Work out the finished part from the listing and answer in its coordinate system (mm). Face numbers are marked on the shaded views. A direction names the side the tool comes from. Give positions to 0.01 mm unless a question says otherwise; leave off trailing zeros. Order: outer loops, then holes, each group sorted by start corner. A loop starts at its lowest first (then second) coordinate and runs counter-clockwise, first axis right, second up. Notation, with made-up numbers: (17, 59.25) - (57, 59.25) arc R29 ccw to (57, 98.25) - close; hole circle Ø8 at (-38, 53). An arc over 180 degrees is marked (long way). Put each result on its own line as item: value.
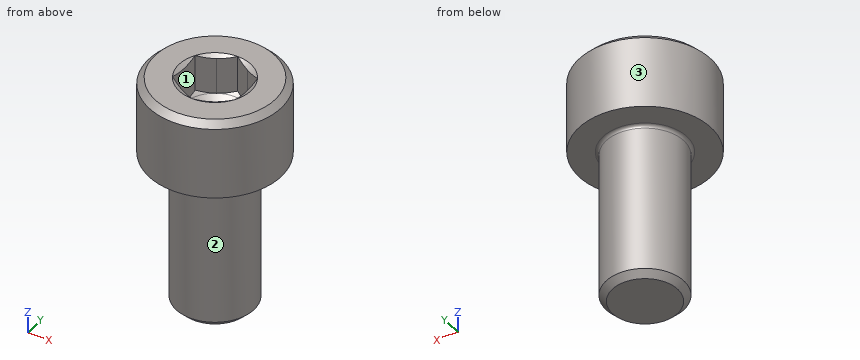
```python
from build123d import *

# Parameters (mm, degrees)
CHAMFER1_SIZE      = 0.4
CUT_EXTRUDE1_START = -2.50000016
CUT_EXTRUDE1_DEPTH = 3.50000016
FILLET2_R          = 0.2


with BuildPart() as part:
    # Sketch1 → Revolve1 (revolve)
    with BuildSketch(Plane(origin=(0, 0, 0), x_dir=(0, 0, -1), z_dir=(1, 0, 0)), mode=Mode.PRIVATE) as revolve1_sk:
        Polygon((0, 4.25), (-5, 4.25), (-5, 0), (10, 0), (10, 2.5), (0, 2.5), align=None)
    revolve(revolve1_sk.sketch.rotate(Axis((0, 0, 5), (0, 0, -1)), 180), axis=Axis((0, 0, 5), (0, 0, -1)))

    # Sketch7 → Cut-Revolve2 (revolve, cut)
    with BuildSketch(Plane(origin=(0, 0, 0), x_dir=(0, 0, -1), z_dir=(1, 0, 0)), mode=Mode.PRIVATE) as cut_revolve2_sk:
        Polygon((-5, 0), (-5, 2), (-2.5, 2), (-1.345299462, 0), align=None)
    revolve(cut_revolve2_sk.sketch.rotate(Axis((0, 0, 5), (0, 0, -1)), 90), axis=Axis((0, 0, 5), (0, 0, -1)), mode=Mode.SUBTRACT)

    # Chamfer1
    chamfer1_edges = [part.edges().sort_by_distance(p)[0] for p in [
        (0, 4.25, 5),
        (0, 2.5, -10),
    ]]
    chamfer(chamfer1_edges, length=CHAMFER1_SIZE)

    # Cut-Extrude1: read off the stored shape, not the designer's step
    # Cut-Extrude1 outline → Cut-Extrude1 (cut)
    with BuildSketch(Plane.XY.offset(5).offset(CUT_EXTRUDE1_START)):
        with BuildLine():
            Line((2, 0), (2, 1.154700538))
            Line((2, 1.154700538), (1.000013378, 1.732043084))
            ThreePointArc((1.000013378, 1.732043084), (1.732054669, 0.999993311), (2, 0))
        make_face()
        with BuildLine():
            ThreePointArc((-1.000013378, 1.732043084), (0, 2), (1.000013378, 1.732043084))
            Line((1.000013378, 1.732043084), (0, 2.309401077))
            Line((0, 2.309401077), (-1.000013378, 1.732043084))
        make_face()
        with BuildLine():
            Line((2, -1.154700538), (2, 0))
            ThreePointArc((2, 0), (1.732054669, -0.999993311), (1.000013378, -1.732043084))
            Line((1.000013378, -1.732043084), (2, -1.154700538))
        make_face()
        with BuildLine():
            ThreePointArc((-2, 0), (-1.732054669, 0.999993311), (-1.000013378, 1.732043084))
            Line((-1.000013378, 1.732043084), (-2, 1.154700538))
            Line((-2, 1.154700538), (-2, 0))
        make_face()
        with BuildLine():
            Line((0, -2.309401077), (1.000013378, -1.732043084))
            ThreePointArc((1.000013378, -1.732043084), (0, -2), (-1.000013377, -1.732043084))
            Line((-1.000013377, -1.732043084), (0, -2.309401077))
        make_face()
        with BuildLine():
            ThreePointArc((-1.000013377, -1.732043084), (-1.732054669, -0.999993311), (-2, 0))
            Line((-2, 0), (-2, -1.154700538))
            Line((-2, -1.154700538), (-1.000013377, -1.732043084))
        make_face()
    extrude(amount=CUT_EXTRUDE1_DEPTH, mode=Mode.SUBTRACT)

    # Cut-Extrude1 2 outline → Cut-Extrude1 2 (revolve)
    with BuildSketch(Plane.XZ):
        Polygon((2.309401238, 2.678632888), (1.999999931, 2.49999996), (2.309401077, 2.49999984), align=None)
    revolve(axis=Axis((0, 0, 0), (0, 0, 1)))

    # Sketch9 → Cut-Revolve3 (revolve, cut)
    with BuildSketch(Plane(origin=(0, 0, 0), x_dir=(0, 0, -1), z_dir=(1, 0, 0))):
        Polygon((-5.5, 3.175426481), (-5.5, 2), (-4.821367205, 2), align=None)
    revolve(axis=Axis((0, 0, 5), (0, 0, -1)), mode=Mode.SUBTRACT)

    # Fillet2
    fillet2_edges = [part.edges().sort_by_distance(p)[0] for p in [
        (0, 2.5, 0),
    ]]
    fillet(fillet2_edges, radius=FILLET2_R)


solid = part.part
```
(1) Section A-A, the plane z = -2.5 is taken. Write down the section's boundary in (x, y), then the cut area to 3 significant figures.
Geometry check:
outline: circle Ø5 at (0, 0)
area: 19.6 mm²
(2) Section B-B, the plane z = 2 is taken. Write down the section's boundary in (x, y), then the cut area to 3 significant figures.
Geometry check:
outline: circle Ø8.5 at (0, 0); hole circle Ø2.27 at (0, 0)
area: 52.7 mm²
(3) Straight lines are drawn through the part: line 1 (Z direction, x = 2, y = 3.25); line 2 (Y direction, x = 1.5, z = -2.5); line 3 (Y direction, x = 0.75, z = 2). For each, find the intervals that lie inside material, in ascending order.
Geometry check:
line 1: z = 0 to 5
line 2: y = -2 to 2
line 3: y = -4.18 to -0.85, 0.85 to 4.18
(4) A tool of negligible diameter and unlimited length cuts with its end or side. For the marked faces 1, 2 and 3, from which of +Z, -Z, +X, -X, +Y, -Y can it reach the whole face along a straight path? Write none if from no direction.
Geometry check:
face 1: +Z
face 2: -Z
face 3: +Z, -Z
(5) Given pin 1 (1 mm diameter, centred on y = 2.5, z = -8.5, fed in from +X); pin 2 (4 mm diameter, centred on x = -3.5, z = 1, fed in from +Y); pin 3 (1 mm diameter, centred on x = 0, z = -3.5, fed in from +Y), each flat-ended and moving along its own axis, determine where each tip first touches the part or whether it passes through.
Geometry check:
pin 1: stops at x = 1.5
pin 2: stops at y = 3.98
pin 3: stops at y = 2.5
